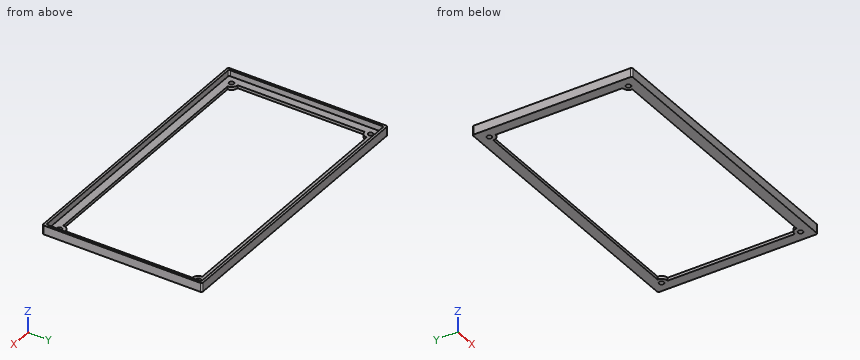
from build123d import *

# Parameters (mm, degrees)
SKETCH_1_W      = 185.6
SKETCH_1_H      = 103.6
SKETCH_1_R      = 1.6
EXTRUDE_1_DEPTH = 2
SKETCH_1_3_W    = 188.8
SKETCH_1_3_H    = 106.8
SKETCH_1_3_W_2  = 185.6
SKETCH_1_3_H_2  = 103.6
EXTRUDE_2_DEPTH = 6
FILLET_1_R      = 1


with BuildPart() as part:
    # Эскиз1 → Бобышка-Вытянуть1 (new body)
    with BuildSketch(Plane.XY):
        with Locations((94.4, 53.4)):
            Rectangle(SKETCH_1_W, SKETCH_1_H)
        with BuildLine():
            ThreePointArc((177.9, 99.9), (179.071572875, 97.071572875), (181.9, 95.9))
            Line((181.9, 95.9), (181.9, 10.9))
            ThreePointArc((181.9, 10.9), (179.071572875, 9.728427125), (177.9, 6.9))
            Line((177.9, 6.9), (10.9, 6.9))
            ThreePointArc((10.9, 6.9), (9.728427125, 9.728427125), (6.9, 10.9))
            Line((6.9, 10.9), (6.9, 95.9))
            ThreePointArc((6.9, 95.9), (9.728427125, 97.071572875), (10.9, 99.9))
            Line((10.9, 99.9), (177.9, 99.9))
        make_face(mode=Mode.SUBTRACT)
        with Locations((181.9, 99.9)):
            Circle(SKETCH_1_R, mode=Mode.SUBTRACT)
        with Locations((181.9, 6.9)):
            Circle(SKETCH_1_R, mode=Mode.SUBTRACT)
        with Locations((6.9, 99.9)):
            Circle(SKETCH_1_R, mode=Mode.SUBTRACT)
        with Locations((6.9, 6.9)):
            Circle(SKETCH_1_R, mode=Mode.SUBTRACT)
    extrude(amount=EXTRUDE_1_DEPTH)

    # Эскиз1<3> → Бобышка-Вытянуть2 (add)
    with BuildSketch(Plane.XY):
        with Locations((94.4, 53.4)):
            Rectangle(SKETCH_1_3_W, SKETCH_1_3_H)
        with Locations((94.4, 53.4)):
            Rectangle(SKETCH_1_3_W_2, SKETCH_1_3_H_2, mode=Mode.SUBTRACT)
    extrude(amount=EXTRUDE_2_DEPTH)

    # Скругление1
    fillet_1_edges = [part.edges().sort_by_distance(p)[0] for p in [
        (0, 0, 3),
        (188.8, 0, 3),
        (188.8, 106.8, 3),
        (187.2, 105.2, 4),
        (187.2, 1.6, 4),
        (1.6, 1.6, 4),
        (1.6, 105.2, 4),
        (0, 106.8, 3),
    ]]
    fillet(fillet_1_edges, radius=FILLET_1_R)


solid = part.part
Read the model definition and answer for the solid it produces. Units are mm, in the model's axes. Give positions to 0.01 mm unless a question says otherwise; leave off trailing zeros. Write each loop counter-clockwise with the first axis right and the second up, starting at its lowest first coordinate (ties: lowest second). Pieces come first, ordered by that corner, then holes. Notation, with made-up numbers: M 70,-37.5 L 80,-37.5 A24 cw 80,-12.5 Z; hole C -16,21.25 d2. An arc over 180 degrees is marked long. One line per item, written item: value. Start each with the question number.
(1) Find section C-C (z = 3.2). Determine the outline of the cut face in (x, y), plus the area to 3 significant figures.
(2) Find section A-A (y = 43). Determine the outline of the cut face in (x, z).
(3) A flat-ended cylindrical pin translates along its axis: pin 1 Ø3.5 at (x, y) = (6.9, 99.9) entering from +Z. Find the tip coordinate at first contact, or state that the pin passes through.
(4) Find section B-B (x = 173.5). Determine the outline of the cut face in (y, z), plus the area to 3 significant figures.
(5) Find the intervals of material crossed by line 1 (X direction, y = 100.5, z = 3.2); line 2 (Y direction, x = 170, z = 2.25); line 3 (X direction, y = 59, z = 0.55), in increasing order.
Results below:
1. outline: M 0,1 A1 ccw 1,0 L 187.8,0 A1 ccw 188.8,1 L 188.8,105.8 A1 ccw 187.8,106.8 L 1,106.8 A1 ccw 0,105.8 Z; hole M 1.6,2.6 A1 ccw 2.6,1.6 L 186.2,1.6 A1 ccw 187.2,2.6 L 187.2,104.2 A1 ccw 186.2,105.2 L 2.6,105.2 A1 ccw 1.6,104.2 Z
1. area: 936 mm^2
2. outline: M 0,0 L 6.9,0 L 6.9,2 L 1.6,2 L 1.6,6 L 0,6 Z; M 181.9,0 L 188.8,0 L 188.8,6 L 187.2,6 L 187.2,2 L 181.9,2 Z
3. pin 1: stops at z = 2
4. outline: M 0,0 L 6.9,0 L 6.9,2 L 1.6,2 L 1.6,6 L 0,6 Z; M 99.9,0 L 106.8,0 L 106.8,6 L 105.2,6 L 105.2,2 L 99.9,2 Z
4. area: 40.4 mm^2
5. line 1: x = 0 to 1.6, 187.2 to 188.8
5. line 2: y = 0 to 1.6, 105.2 to 106.8
5. line 3: x = 0 to 6.9, 181.9 to 188.8
